Check sheet for the modelled part. Datum: model origin and axes. Units: mm. Face numbers are marked on the shaded views. A direction names the side the tool comes from. Give positions to 0.01 mm unless a question says otherwise; leave off trailing zeros. Order: outer loops, then holes, each group sorted by start corner. A loop starts at its lowest first (then second) coordinate and runs counter-clockwise, first axis right, second up.
```python
from build123d import *

# Parameters (mm, degrees)
SKETCH1_W           = 90
SKETCH1_H           = 45
BOSS_EXTRUDE1_DEPTH = 50
SHELL1_T            = -2.5
SKETCH2_W           = 40
SKETCH2_H           = 24.5
BOSS_EXTRUDE2_DEPTH = 10
SKETCH3_W           = 40
SKETCH3_H           = 19.5
BOSS_EXTRUDE3_DEPTH = 10
SKETCH9_W           = 20
SKETCH9_H           = 10
CUT_EXTRUDE3_DEPTH  = 2.5
SKETCH13_W          = 40
SKETCH13_H          = 5
CUT_EXTRUDE6_DEPTH  = 2.5
SKETCH14_W          = 87.5
SKETCH14_H          = 2
CUT_EXTRUDE7_DEPTH  = 1
SKETCH15_W          = 87.5
SKETCH15_H          = 2
CUT_EXTRUDE8_DEPTH  = 1
SKETCH17_R          = 1.5
CUT_EXTRUDE9_DEPTH  = 27
SKETCH18_R          = 1.5
CUT_EXTRUDE10_DEPTH = 27
SKETCH20_R          = 1.5
CUT_EXTRUDE11_DEPTH = 22
SKETCH21_R          = 1.5
CUT_EXTRUDE12_DEPTH = 22
SKETCH22_R          = 3
CUT_EXTRUDE13_DEPTH = 5
SKETCH26_W          = 15
SKETCH26_H          = 15
CUT_EXTRUDE14_DEPTH = 12.5


with BuildPart() as part:
    # Sketch1 → Boss-Extrude1 (new body)
    with BuildSketch(Plane(origin=(0, 0, 0), x_dir=(1, 0, 0), z_dir=(0, 1, 0))):
        with Locations((4.862356655, 3.4550978)):
            Rectangle(SKETCH1_W, SKETCH1_H)
    extrude(amount=BOSS_EXTRUDE1_DEPTH)

    # Shell1
    shell1_openings = [part.faces().sort_by_distance(p)[0] for p in [
        (4.862356655, 50, -3.4550978),
    ]]
    offset(amount=SHELL1_T, openings=shell1_openings, kind=Kind.INTERSECTION)

    # Sketch2 → Boss-Extrude2 (add)
    with BuildSketch(Plane(origin=(-37.637643345, 0, 0), x_dir=(0, 0, -1), z_dir=(1, 0, 0))):
        with Locations((3.4550978, 14.75)):
            Rectangle(SKETCH2_W, SKETCH2_H)
    extrude(amount=BOSS_EXTRUDE2_DEPTH)

    # Sketch3 → Boss-Extrude3 (add)
    with BuildSketch(Plane.ZY.offset(-47.362356655)):
        with Locations((-3.4550978, 12.25)):
            Rectangle(SKETCH3_W, SKETCH3_H)
    extrude(amount=BOSS_EXTRUDE3_DEPTH)

    # Sketch9 → Cut-Extrude3 (cut)
    with BuildSketch(Plane(origin=(-37.637643345, 0, 0), x_dir=(0, 0, -1), z_dir=(1, 0, 0))):
        with Locations((3.4550978, 32)):
            Rectangle(SKETCH9_W, SKETCH9_H)
    extrude(amount=-CUT_EXTRUDE3_DEPTH, mode=Mode.SUBTRACT)

    # Sketch13 → Cut-Extrude6 (cut)
    with BuildSketch(Plane(origin=(-37.637643345, 0, 0), x_dir=(0, 0, -1), z_dir=(1, 0, 0))):
        with Locations((3.4550978, 47.5)):
            Rectangle(SKETCH13_W, SKETCH13_H)
    extrude(amount=-CUT_EXTRUDE6_DEPTH, mode=Mode.SUBTRACT)

    # Sketch14 → Cut-Extrude7 (cut)
    with BuildSketch(Plane.XY.offset(-23.4550978)):
        with Locations((3.612356655, 46)):
            Rectangle(SKETCH14_W, SKETCH14_H)
    extrude(amount=-CUT_EXTRUDE7_DEPTH, mode=Mode.SUBTRACT)

    # Sketch15 → Cut-Extrude8 (cut)
    with BuildSketch(Plane(origin=(0, 0, 16.5449022), x_dir=(-1, 0, 0), z_dir=(0, 0, -1))):
        with Locations((-3.612356655, 46)):
            Rectangle(SKETCH15_W, SKETCH15_H)
    extrude(amount=-CUT_EXTRUDE8_DEPTH, mode=Mode.SUBTRACT)

    # Sketch17 → Cut-Extrude9 (cut)
    with BuildSketch(Plane(origin=(0, 27, 0), x_dir=(1, 0, 0), z_dir=(0, 1, 0))):
        with Locations(Location((-32.637643345, -9.0449022, 0), (0, 0, 270))):
            Circle(SKETCH17_R)
    extrude(amount=-CUT_EXTRUDE9_DEPTH, mode=Mode.SUBTRACT)

    # Sketch18 → Cut-Extrude10 (cut)
    with BuildSketch(Plane(origin=(0, 27, 0), x_dir=(1, 0, 0), z_dir=(0, 1, 0))):
        with Locations(Location((-32.637643345, 15.9550978, 0), (0, 0, 270))):
            Circle(SKETCH18_R)
    extrude(amount=-CUT_EXTRUDE10_DEPTH, mode=Mode.SUBTRACT)

    # Sketch20 → Cut-Extrude11 (cut)
    with BuildSketch(Plane(origin=(0, 22, 0), x_dir=(1, 0, 0), z_dir=(0, 1, 0))):
        with Locations(Location((42.362356655, 15.9550978, 0), (0, 0, 270))):
            Circle(SKETCH20_R)
    extrude(amount=-CUT_EXTRUDE11_DEPTH, mode=Mode.SUBTRACT)

    # Sketch21 → Cut-Extrude12 (cut)
    with BuildSketch(Plane(origin=(0, 22, 0), x_dir=(1, 0, 0), z_dir=(0, 1, 0))):
        with Locations(Location((42.362356655, -9.0449022, 0), (0, 0, 270))):
            Circle(SKETCH21_R)
    extrude(amount=-CUT_EXTRUDE12_DEPTH, mode=Mode.SUBTRACT)

    # Sketch22 → Cut-Extrude13 (cut)
    with BuildSketch(Plane.XZ):
        with Locations(Location((-32.637643345, -15.9550978, 0), (0, 0, 270))):
            Circle(SKETCH22_R)
        with Locations(Location((-32.637643345, 9.0449022, 0), (0, 0, 270))):
            Circle(SKETCH22_R)
        with Locations(Location((42.362356655, -15.9550978, 0), (0, 0, 270))):
            Circle(SKETCH22_R)
        with Locations(Location((42.362356655, 9.0449022, 0), (0, 0, 270))):
            Circle(SKETCH22_R)
    extrude(amount=-CUT_EXTRUDE13_DEPTH, mode=Mode.SUBTRACT)

    # Sketch26 → Cut-Extrude14 (cut)
    with BuildSketch(Plane.ZY.offset(-37.362356655)):
        with Locations((-3.4550978, 10)):
            Rectangle(SKETCH26_W, SKETCH26_H)
    extrude(amount=-CUT_EXTRUDE14_DEPTH, mode=Mode.SUBTRACT)


solid = part.part
```
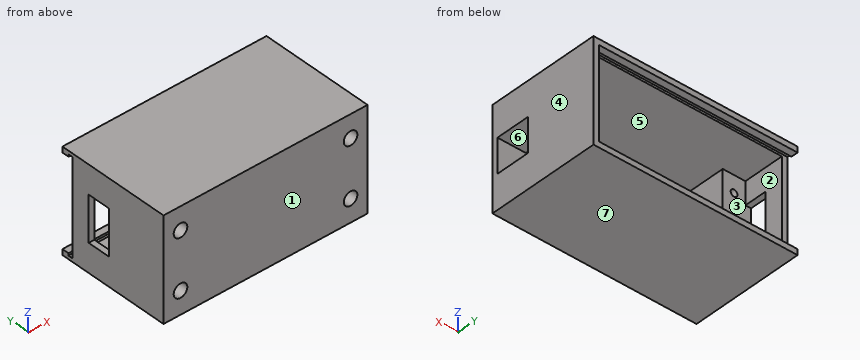
(1) Cross-section at C-C on z = 14. Enter the section's corners in (x, y), then the cut area to 3 significant figures.
Response values:
outline: (-40.14, 0) - (49.86, 0) - (49.86, 50) - (47.36, 50) - (47.36, 22) - (37.36, 22) - (37.36, 2.5) - (-27.64, 2.5) - (-27.64, 27) - (-37.64, 27) - (-37.64, 45) - (-40.14, 45) - close
area: 890 mm2
(2) Set-up check for the marked faces 5, 6 and 7: record each of +Z, -Z, +X, -X, +Y, -Y from which the full face is reachable in a straight line by a thin tool's end or side.
Response values:
face 5: +Y
face 6: +X
face 7: -Z, +X, -X, +Y, -Y
(3) Cross-section at A-A on z = -5. Enter the section's corners in (x, y), then the cut area to 4 significant figures.
Response values:
outline: (-40.14, 0) - (49.86, 0) - (49.86, 2.5) - (-27.64, 2.5) - (-27.64, 27) - (-40.14, 27) - close; (-40.14, 37) - (-37.64, 37) - (-37.64, 45) - (-40.14, 45) - close; (37.36, 17.5) - (49.86, 17.5) - (49.86, 50) - (47.36, 50) - (47.36, 22) - (37.36, 22) - close
area: 677.5 mm2
(4) Gauge pin test, flat ends, axial feed: pin 1 Ø7 at (x, z) = (42.36, 9.04) entering from +Y; pin 2 Ø3 at (x, z) = (-8.5, -4) entering from +Y; pin 3 Ø1.8 at (x, z) = (-32.5, -15) entering from -Y. Record the tip position at first contact, or that the pin passes through.
Response values:
pin 1: stops at y = 22
pin 2: stops at y = 2.5
pin 3: stops at y = 5
(5) Release check for a two-part mould opening along X. For the marked faces 1, 2, 3 and 4 record: released by +X, released by -X, zero draft, split by the parting line, or undercut.
Response values:
face 1: zero draft
face 2: undercut
face 3: undercut
face 4: released by +X
(6) Material ranges on L1, parallel to Z at x = 20.5, y = 3.5; L2, parallel to X at y = 39.5, z = -5; L3, parallel to Z at x = -34, y = 46.5, recorded low to high.
Response values:
L1: z = -25.96 to -23.46, 16.54 to 19.04
L2: x = -40.14 to -37.64, 47.36 to 49.86
L3: z = -25.96 to -24.46, 17.54 to 19.04
(7) Cross-section at B-B on y = 41. Enter the section's corners in (x, z), then the cut area to 3 significant figures.
Response values:
outline: (-40.14, -25.96) - (49.86, -25.96) - (49.86, 19.04) - (-40.14, 19.04) - close; hole (-37.64, -23.46) - (47.36, -23.46) - (47.36, 16.54) - (-37.64, 16.54) - close
area: 650 mm2
(8) Cross-section at D-D on x = -6. Enter the section's corners in (y, z).
Response values:
outline: (0, -25.96) - (50, -25.96) - (50, -23.46) - (47, -23.46) - (47, -24.46) - (45, -24.46) - (45, -23.46) - (2.5, -23.46) - (2.5, 16.54) - (45, 16.54) - (45, 17.54) - (47, 17.54) - (47, 16.54) - (50, 16.54) - (50, 19.04) - (0, 19.04) - close
